```python
from build123d import *

# Parameters (mm, degrees)
SZKIC1_W                      = 30
SZKIC1_H                      = 3.15
DODANIE_WYCI_GNI_CIE1_DEPTH   = 15
DODANIE_WYCI_GNI_CIE1_2_DEPTH = 15
DODANIE_WYCI_GNI_CIE1_3_DEPTH = 15
DODANIE_WYCI_GNI_CIE2_DEPTH   = 2
ZAOKR_GLENIE1_R               = 10
ZAOKR_GLENIE2_R               = 2


with BuildPart() as part:
    # Szkic1 → Dodanie-wyci_gni_cie1 (new body)
    with BuildSketch(Plane.XY):
        with Locations((0, 4.675)):
            Rectangle(SZKIC1_W, SZKIC1_H)
    extrude(amount=DODANIE_WYCI_GNI_CIE1_DEPTH)



with BuildPart() as body_2:
    # Szkic1 → Dodanie-wyci_gni_cie1 2 (new body)
    with BuildSketch(Plane.XY):
        Polygon((-15, -6.25), (-5, -30), (-3.1, -30), (-3.1, -3.1), (-15, -3.1), align=None)
    extrude(amount=DODANIE_WYCI_GNI_CIE1_2_DEPTH)


with BuildPart() as body_3:
    # Szkic1 → Dodanie-wyci_gni_cie1 3 (new body)
    with BuildSketch(Plane.XY):
        Polygon((3.1, -3.1), (3.1, -30), (5, -30), (15, -6.25), (15, -3.1), align=None)
    extrude(amount=DODANIE_WYCI_GNI_CIE1_3_DEPTH)


with BuildPart() as part_1:
    add(part.part)

    add(body_2.part)  # Dodanie-wyci_gni_cie2 merges body 2

    add(body_3.part)  # Dodanie-wyci_gni_cie2 merges body 3
    # Szkic1_3 → Dodanie-wyci_gni_cie2 (add)
    with BuildSketch(Plane.XY):
        Polygon((-5, -30), (5, -30), (15, -6.25), (15, 6.25), (-15, 6.25), (-15, -6.25), align=None)
    extrude(amount=-DODANIE_WYCI_GNI_CIE2_DEPTH)

    # Zaokr_glenie1
    zaokr_glenie1_edges = [part_1.edges().sort_by_distance(p)[0] for p in [
        (15, -6.25, 6.5),
        (-15, -6.25, 6.5),
    ]]
    fillet(zaokr_glenie1_edges, radius=ZAOKR_GLENIE1_R)

    # Zaokr_glenie2
    zaokr_glenie2_edges = [part_1.edges().sort_by_distance(p)[0] for p in [
        (5, -30, 6.5),
        (-5, -30, 6.5),
        (-15, 6.25, 6.5),
        (15, 6.25, 6.5),
    ]]
    fillet(zaokr_glenie2_edges, radius=ZAOKR_GLENIE2_R)


solid = part_1.part
```
The listing builds one solid part. Answer for the finished solid, in the listing's coordinates (mm). A direction names the side the tool comes from. Give positions to 0.01 mm unless a question says otherwise; leave off trailing zeros. Order: outer loops, then holes, each group sorted by start corner. A loop starts at its lowest first (then second) coordinate and runs counter-clockwise, first axis right, second up. Notation, with made-up numbers: (68, 87) -> (97, 87) arc R16 ccw to (97, 113) -> close; hole circle Ø10 at (13.25, 76.25). An arc over 180 degrees is marked (long way). Answer as a JSON object with one key per item and string values. Group by question number.
Item 1: The part is cut by section C-C on x = -5. Write down the section's boundary in (y, z).
Item 2: Determine the mould class of faces 1 (the flat face through (-9, -3.1, 7)), 2 (the cylindrical face through (14.81, -6.18, 6.62)), 3 (the flat face through (9, -3.1, 7)), 4 (the flat face through (0, -8, -2)) for opening direction Y: pulls with the +Y half, pulls with the -Y half, needs draft (parallel to the pull), parting line crosses it, or undercut.
Item 3: A tool of negligible diameter and unlimited length cuts with its end or side. For faces 5 (the flat face through (-3.1, -17, 7)), 6 (the flat face through (0, 3.1, 7)), 7 (the flat face through (0, 6.25, 7)), from which of +Z, -Z, +X, -X, +Y, -Y can it reach the whole face along a straight path? Write none if from no direction.
Item 4: The part is cut by section B-B on y = -20.5. Write down the section's boundary in (x, z), and give its area (3 significant figures).
Item 5: Consider L1, parallel to Z at x = -1.25, y = 1; L2, parallel to X at y = -27.5, z = 11.75; L3, parallel to X at y = -17, z = 7. Determine where each line is inside the solid, lowest interval first. Write a range as from..to.
Item 6: The part is cut by section D-D on x = 2.5. Write down the section's boundary in (y, z), and give its area (3 significant figures).
Item 7: The part is cut by section A-A on z = 13.5. Write down the section's boundary in (x, y).
Item 8: Flat-ended cylindrical pins translate along their axes: pin 1 (4.5 mm diameter, centred on y = -17.5, z = 4.5, fed in from -X); pin 2 (6 mm diameter, centred on x = -11, z = 3, fed in from -Y) (3 decimals); pin 3 (4 mm diameter, centred on y = -23, z = 10, fed in from -X). Find the tip coordinate at first contact, or state that the pin passes through.
Result set:
{
 "1": {"outline": "(-29.5, -2) -> (6.25, -2) -> (6.25, 15) -> (3.1, 15) -> (3.1, 0) -> (-3.1, 0) -> (-3.1, 15) -> (-29.5, 15) -> close"},
 "2": {"face 1": "undercut", "face 2": "pulls with the -Y half", "face 3": "undercut", "face 4": "needs draft"},
 "3": {"face 5": "+Z, -Y", "face 6": "+Z, +X, -X", "face 7": "+Z, -Z, +X, -X, +Y"},
 "4": {"outline": "(-9, -2) -> (9, -2) -> (9, 15) -> (3.1, 15) -> (3.1, 0) -> (-3.1, 0) -> (-3.1, 15) -> (-9, 15) -> close", "area": "213 mm²"},
 "5": {"L1": "-2..0", "L2": "-6.05..-3.1, 3.1..6.05", "L3": "-10.47..-3.1, 3.1..10.47"},
 "6": {"outline": "(-30, -2) -> (6.25, -2) -> (6.25, 15) -> (3.1, 15) -> (3.1, 0) -> (-30, 0) -> close", "area": "120 mm²"},
 "7": {"outline": "(-15, -4.23) arc R10 ccw to (-14.22, -8.11) -> (-5.52, -28.78) arc R2 ccw to (-3.67, -30) -> (-3.1, -30) -> (-3.1, -3.1) -> (-15, -3.1) -> close; (-15, 3.1) -> (15, 3.1) -> (15, 4.25) arc R2 ccw to (13, 6.25) -> (-13, 6.25) arc R2 ccw to (-15, 4.25) -> close; (3.1, -30) -> (3.67, -30) arc R2 ccw to (5.52, -28.78) -> (14.22, -8.11) arc R10 ccw to (15, -4.23) -> (15, -3.1) -> (3.1, -3.1) -> close"},
 "8": {"pin 1": "x = -11.21", "pin 2": "y = -22.875", "pin 3": "x = -8.79"}
}
